Model file for the job. Use its own axes, mm. Face numbers are marked on the shaded views. Coordinates: 2 decimals unless noted, no trailing zeros. Order: outer loops, then holes, each group sorted by start corner. A loop starts at its lowest first (then second) coordinate and runs counter-clockwise, first axis right, second up. Notation, with made-up numbers: (-1, 80.5) -> (21, 80.5) arc R17 cw to (21, 84.5) -> close; hole circle Ø8 at (-19.5, 32). An arc over 180 degrees is marked (long way). Return JSON: item names as keys, results as strings. Group by question number.
1) Cut at A-A (y = -4.2). Write the cut outline in (x, z), and give its area (3 significant figures).
2) Flat gauge pin, fed straight in: pin 1 (1.5 mm diameter, centred on x = -0.5, y = -3.5, fed in from -Z). Where does the tip first touch, or does it go through?
3) Pull direction X, two halves, no side cores. Call the marked faces 1, 2 and 3: +X half, -X half, draft (parallel to the pull), parting line (faces both ways), or undercut.
4) Cut at D-D (z = 4.5). Write the cut outline in (x, y), and give its area (3 significant figures).
5) Cut at B-B (z = 0). Write the cut outline in (x, y).
6) Probe line 1 (Z direction, x = -1.75, y = -1.7); line 2 (Z direction, x = 0.75, y = -2.3); line 3 (X direction, y = -0.2, z = 2). List the from-to ranges inside material, lowest first.
7) Cut at C-C (x = 0.5). Write the cut outline in (y, z), and give its area (3 significant figures).
Solid Edge part; units mm, degrees
sketch "Sketch1" plane through (0, 0, 0) normal (0, -1, 0) x (1, 0, 0)
  circle A0 centre (0, 0) radius 3
  line L0 (5, 2.8868) -> (0, 5.7735)
  line L1 (0, 5.7735) -> (-5, 2.8868)
  line L2 (-5, 2.8868) -> (-5, -2.8868)
  line L3 (-5, -2.8868) -> (0, -5.7735)
  line L4 (0, -5.7735) -> (5, -2.8868)
  line L5 (5, -2.8868) -> (5, 2.8868)
extrude "Protrusion1" add sketch "Sketch1" along normal blind 5
cosmetic_thread "Thread1"
properties material "NYLON"
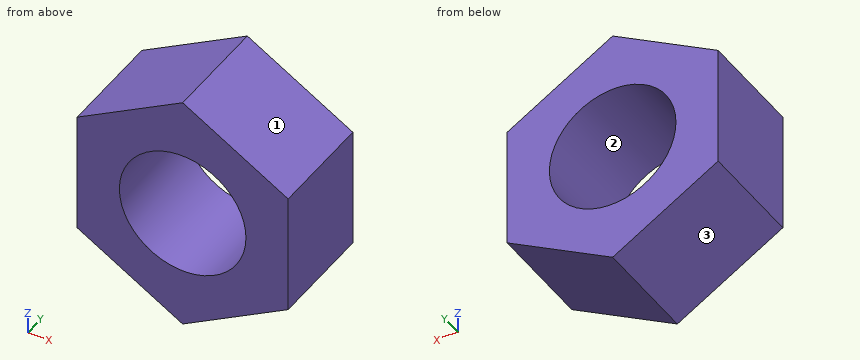
Answers below:
{
 "1": {"outline": "(-5, -2.89) -> (0, -5.77) -> (5, -2.89) -> (5, 2.89) -> (0, 5.77) -> (-5, 2.89) -> close; hole circle Ø6 at (0, 0)", "area": "58.3 mm^2"},
 "2": {"pin 1": "stops at z = -5.77"},
 "3": {"face 1": "+X half", "face 2": "undercut", "face 3": "-X half"},
 "4": {"outline": "(-2.21, -5) -> (2.21, -5) -> (2.21, 0) -> (-2.21, 0) -> close", "area": "22.1 mm^2"},
 "5": {"outline": "(-5, -5) -> (-3, -5) -> (-3, 0) -> (-5, 0) -> close; (3, -5) -> (5, -5) -> (5, 0) -> (3, 0) -> close"},
 "6": {"line 1": "z = -4.76 to -2.44, 2.44 to 4.76", "line 2": "z = -5.34 to -2.9, 2.9 to 5.34", "line 3": "x = -5 to -2.24, 2.24 to 5"},
 "7": {"outline": "(-5, -5.48) -> (0, -5.48) -> (0, -2.96) -> (-5, -2.96) -> close; (-5, 2.96) -> (0, 2.96) -> (0, 5.48) -> (-5, 5.48) -> close", "area": "25.3 mm^2"}
}
